from build123d import *

# Parameters (mm, degrees)
F0_R     = 35
F0_R_2   = 10
F1_DEPTH = 25
F2_R     = 35
F2_R_2   = 27.5
F3_DEPTH = 20
F4_W     = 13.364931
F4_H     = 62.559245
F5_DEPTH = 25


with BuildPart() as f1:
    # F0 (on Front) → F1 (new body)
    with BuildSketch(Plane.XZ):
        Circle(F0_R)
        Circle(F0_R_2, mode=Mode.SUBTRACT)
    extrude(amount=F1_DEPTH)

    # F2 (on face) → F3 (cut)
    with BuildSketch(Plane(origin=(0, 0, 0), x_dir=(-1, 0, 0), z_dir=(0, 1, 0))):
        Circle(F2_R)
        Circle(F2_R_2, mode=Mode.SUBTRACT)
    extrude(amount=-F3_DEPTH, mode=Mode.SUBTRACT)

    # F4 (on face) → F5 (cut)
    with BuildSketch(Plane.XZ.offset(25)):
        with Locations((-36.682465, -1.913552)):
            Rectangle(F4_W, F4_H)
        with Locations((36.682465, -1.913552)):
            Rectangle(F4_W, F4_H)
    extrude(amount=-F5_DEPTH, mode=Mode.SUBTRACT)


solid = f1.part
Read the model definition and answer for the solid it produces. Units are mm, in the model's axes. A direction names the side the tool comes from. Give positions to 0.01 mm unless a question says otherwise; leave off trailing zeros. Write each loop counter-clockwise with the first axis right and the second up, starting at its lowest first coordinate (ties: lowest second). Pieces come first, ordered by that corner, then holes. Notation, with made-up numbers: (62, 40) - (87, 40) arc R33 cw to (87, 73) - close; hole circle Ø9 at (67.5, 54.25). An arc over 180 degrees is marked (long way). Use CSV: the item, a comma, the result in double quotes. Start each with the question number.
Item 1: The part is cut by section A-A, the plane z = 0. Give the vertices of the cut face in (x, y).
Item 2: The part is cut by section C-C, the plane y = -22.5. Give the vertices of the cut face in (x, z).
Item 3: The mould has two halves that part along Z. Classify faces 1 (the cylindrical face through (-0.505, -22.465, -34.996)), 2 (the cylindrical face through (5.961, -9.86, -26.846)), 3 (the cylindrical face through (-2.17, -12.32, -9.76)): pulls with the +Z half, pulls with the -Z half, needs draft (parallel to the pull), parting line crosses it, or undercut.
Item 4: Consider line 1 (Z direction, x = 0, y = -8.75); line 2 (X direction, y = -3.75, z = 7); line 3 (Z direction, x = -8.5, y = -14.5). Determine where each line is inside the solid, lowest interval first.
Item 5: Flat-ended cylindrical pins translate along their axes: P1, Ø6, axis at y = -10.5, z = -19.5, coming from the +X side; P2, Ø18, axis at x = 0, z = 0, coming from the +Y side; P3, Ø5, axis at x = 15.5, y = -15, coming from the -Z side; P4, Ø1.5, axis at x = -21.5, y = -11, coming from the -Z side. Find the tip coordinate at first contact, or state that the pin passes through.
Item 6: The part is cut by section B-B, the plane x = 0. Give the vertices of the cut face in (y, z).
Item 7: For faces 4 (the flat face through (11, -20, -26)), 5 (the flat face through (0, 0, -12)), determine the directions among +Z, -Z, +X, -X, +Y, -Y from which every point of the face is accessible in a straight line to the end or side of a thin tool.
Item 8: The part is cut by section D-D, the plane z = -15. Give the vertices of the cut face in (x, y).
Taken from the geometry:
1,outline,"(-30, -25) - (-10, -25) - (-10, 0) - (-27.5, 0) - (-27.5, -20) - (-30, -20) - close; (10, -25) - (30, -25) - (30, -20) - (27.5, -20) - (27.5, 0) - (10, 0) - close"
2,outline,"(-30, -18.03) arc R35 ccw to (30, -18.03) - (30, 18.03) arc R35 ccw to (-30, 18.03) - close; hole circle Ø20 at (0, 0)"
3,face 1,"pulls with the -Z half"
3,face 2,"parting line crosses it"
3,face 3,"undercut"
4,line 1,"-27.5 to -10, 10 to 27.5"
4,line 2,"-26.59 to -7.14, 7.14 to 26.59"
4,line 3,"-26.15 to -5.27, 5.27 to 26.15"
5,P1,"x = 22"
5,P2,"through"
5,P3,"z = -24.23"
5,P4,"z = -18.05"
6,outline,"(-25, -35) - (-20, -35) - (-20, -27.5) - (0, -27.5) - (0, -10) - (-25, -10) - close; (-25, 10) - (0, 10) - (0, 27.5) - (-20, 27.5) - (-20, 35) - (-25, 35) - close"
7,face 4,"+Y"
7,face 5,"+Z, -Z, +X, -X, +Y"
8,outline,"(-30, -25) - (30, -25) - (30, -20) - (23.05, -20) - (23.05, 0) - (-23.05, 0) - (-23.05, -20) - (-30, -20) - close"
